Here's how the part is built. I have some questions about the finished solid (model axes, mm). A direction names the side the tool comes from. Coordinates: 2 decimals unless noted, no trailing zeros. Order: outer loops, then holes, each group sorted by start corner. A loop starts at its lowest first (then second) coordinate and runs counter-clockwise, first axis right, second up. Notation, with made-up numbers: (44.25, 26.25) - (54.25, 26.25) arc R22 ccw to (54.25, 39.25) - close; hole circle Ø7 at (21, 87). An arc over 180 degrees is marked (long way). Answer in a Markdown table with one row per item. Add a question column.
Item 1: On a 3-axis mill with a long thin cutter (end or side, diameter ignored), from which of +Z, -Z, +X, -X, +Y, -Y can I reach the whole of each face in a straight line? I mean faces 1 (the cylindrical face through (-1.38, -6.2, 6.31)), 2 (the flat face through (4, 0, 0)). Say none if no direction works.
Item 2: Will these pins go through, and if not, where does the flat tip stop? pin 1 Ø10 at (x, y) = (-16, -7) entering from +Z (3 decimals); pin 2 Ø3 at (y, z) = (16.5, 1) entering from -X; pin 3 Ø4 at (y, z) = (-2.5, 8) entering from -X.
Item 3: Thinking about a two-plate mould opening in X: for faces 3 (the cylindrical face through (11.52, 18.07, 1.57)), 4 (the cylindrical face through (-1.35, 4.64, 6.29)), 5 (the flat face through (-2, 3, 9.525)), which applies, +X half, -X half, draft (parallel to the pull), parting line (faces both ways), or undercut?
Item 4: I want a section at B-B (x = 0). Please give me the cut outline in (y, z) (3 decimals), plus the area to 3 significant figures.
Item 5: I want a section at D-D (x = 9.5). Please give me the cut outline in (y, z) (3 decimals), plus the area to 3 significant figures.
Item 6: If I drill on line 1 along Z through (x, y) = (0, 5.2) (3 decimals); line 2 along Z through (x, y) = (3, 11) (3 decimals); line 3 along X through (y, z) = (4.3, 6.35), over which ranges is the centre line in solid material (lowest first)? Write a range as from..to.
Item 7: I want a section at A-A (y = 0). Please give me the cut outline in (x, z) (3 decimals), plus the area to 3 significant figures.
```python
from build123d import *

# Parameters (mm, degrees)
SKETCH1_R                  = 21.43125
BOSS_EXTRUDE1_DEPTH        = 3.175
SKETCH2_R                  = 6.35
BOSS_EXTRUDE2_DEPTH        = 6.35
SKETCH3_R                  = 3.175
CUT_EXTRUDE1_DEPTH         = 32.769837553
F_6_32_TAPPED_HOLE1_REACH  = 38.357
F_6_32_TAPPED_HOLE1_BORE_R = 1.35255


with BuildPart() as part:
    # Sketch1 → Boss-Extrude1 (new body)
    with BuildSketch(Plane.XY):
        Circle(SKETCH1_R)
    extrude(amount=BOSS_EXTRUDE1_DEPTH)

    # Sketch2 → Boss-Extrude2 (add)
    with BuildSketch(Plane.XY.offset(3.175)):
        Circle(SKETCH2_R)
    extrude(amount=BOSS_EXTRUDE2_DEPTH)

    # Sketch3 → Cut-Extrude1 (cut, through all)
    with BuildSketch(Plane(origin=(0, 0, 0), x_dir=(-1, 0, 0), z_dir=(0, 0, -1))):
        Circle(SKETCH3_R)
    extrude(amount=-CUT_EXTRUDE1_DEPTH, mode=Mode.SUBTRACT)

    # #6-32 Tapped Hole1 bore → #6-32 Tapped Hole1 (cut, up to next)
    with BuildSketch(Plane(origin=(0, 6.35, 0), x_dir=(1, 0, 0), z_dir=(0, 1, 0)), mode=Mode.PRIVATE) as f_6_32_tapped_hole1_sk1:
        with Locations((0, -6.35)):
            Circle(F_6_32_TAPPED_HOLE1_BORE_R)
    f_6_32_tapped_hole1_tool1 = extrude(f_6_32_tapped_hole1_sk1.sketch, amount=-F_6_32_TAPPED_HOLE1_REACH, mode=Mode.PRIVATE) & part.part
    add(f_6_32_tapped_hole1_tool1.solids().sort_by_distance((0, 6.35, 6.35))[0], mode=Mode.SUBTRACT)


solid = part.part
```
Values follow:
| question | item | result |
|---|---|---|
| 1 | face 1 | +Z |
| 1 | face 2 | -Z, +X, -X, +Y, -Y |
| 2 | pin 1 | stops at z = 3.175 |
| 2 | pin 2 | stops at x = -15.31 |
| 2 | pin 3 | stops at x = -6.33 |
| 3 | face 3 | parting line |
| 3 | face 4 | undercut |
| 3 | face 5 | draft |
| 4 | outline | (-21.431, 0) - (-3.175, 0) - (-3.175, 9.525) - (-6.35, 9.525) - (-6.35, 3.175) - (-21.431, 3.175) - close; (3.175, 0) - (21.431, 0) - (21.431, 3.175) - (6.35, 3.175) - (6.35, 4.997) - (3.175, 4.997) - close; (3.175, 7.703) - (6.35, 7.703) - (6.35, 9.525) - (3.175, 9.525) - close |
| 4 | area | 148 mm^2 |
| 5 | outline | (-19.211, 0) - (19.211, 0) - (19.211, 3.175) - (-19.211, 3.175) - close |
| 5 | area | 122 mm^2 |
| 6 | line 1 | z = 0..4.997, 7.703..9.525 |
| 6 | line 2 | z = 0..3.175 |
| 6 | line 3 | x = -4.67..-1.35, 1.35..4.67 |
| 7 | outline | (-21.431, 0) - (-3.175, 0) - (-3.175, 9.525) - (-6.35, 9.525) - (-6.35, 3.175) - (-21.431, 3.175) - close; (3.175, 0) - (21.431, 0) - (21.431, 3.175) - (6.35, 3.175) - (6.35, 9.525) - (3.175, 9.525) - close |
| 7 | area | 156 mm^2 |
